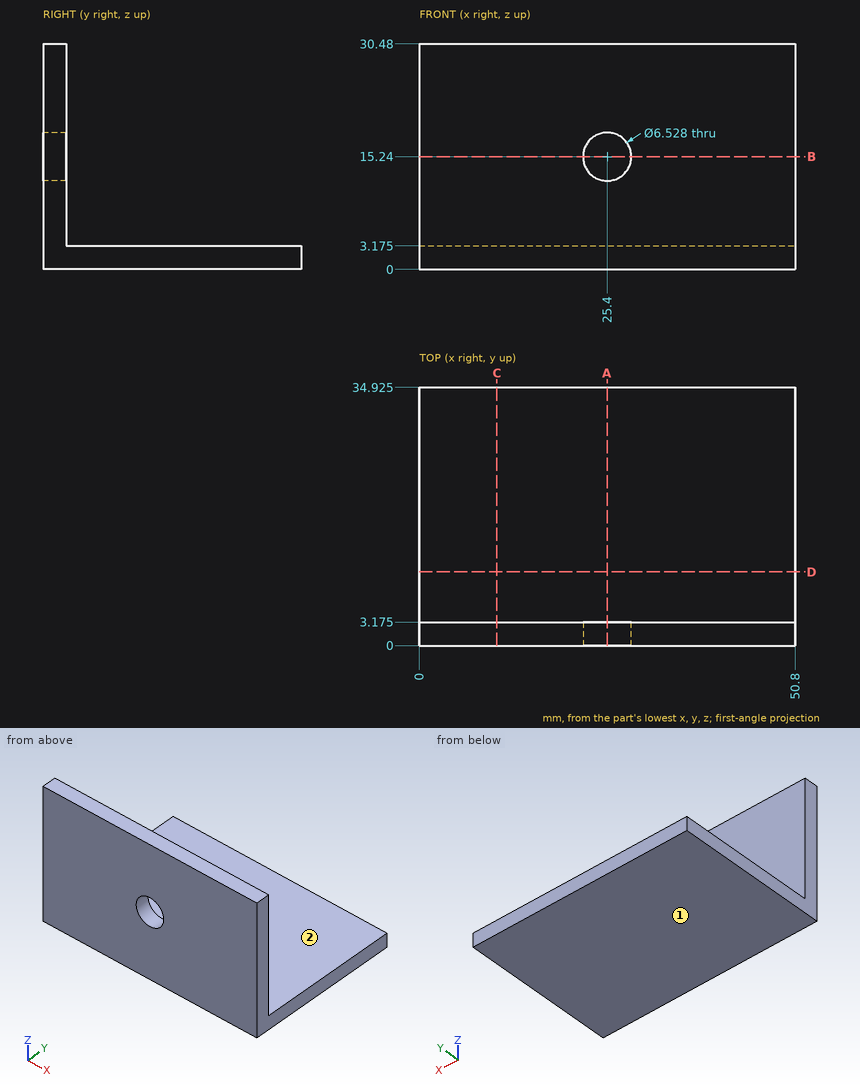
Answer from the drawing. Dimensions are ordinates in mm from the lowest x, y and z of the part. A direction names the side the tool comes from. Give positions to 0.01 mm unless a question says otherwise; leave off trailing zeros. Write each loop counter-clockwise with the first axis right and the second up, starting at its lowest first coordinate (ties: lowest second). Pieces come first, ordered by that corner, then holes. Notation, with made-up numbers: (22, -11) - (81, -11) arc R28 ccw to (81, 7) - close; hole circle Ø7 at (67, -14.75). An arc over 180 degrees is marked (long way). One line per item, written item: value. Start each with the question number.
1. Find section B-B (z = 15.24). Write down the section's boundary in (x, y) (1 decimal).
2. Given pin 1 (4 mm diameter, centred on x = 25.4, z = 15.24, fed in from -Y); pin 2 (2 mm diameter, centred on x = 37, z = 14.5, fed in from +Y) (3 decimals); pin 3 (1.5 mm diameter, centred on x = 19.5, y = 26.5, fed in from +Z) (3 decimals), each flat-ended and moving along its own axis, determine where each tip first touches the part or whether it passes through.
3. Find section C-C (x = 10.5). Write down the section's boundary in (y, z) (3 decimals).
4. Find section D-D (y = 10). Write down the section's boundary in (x, z) (3 decimals), then the cut area to 3 significant figures.
5. For the marked faces 1 and 2, determine the directions among +Z, -Z, +X, -X, +Y, -Y from which every point of the face is accessible in a straight line to the end or side of a thin tool.
6. Find section A-A (x = 25.4). Write down the section's boundary in (y, z) (1 decimal), then the cut area to 3 significant figures.
7. Consider probe 1 along Z at (x, y) = (25.4, 2.15); probe 2 along X at (y, z) = (2, 15) (1 decimal); probe 3 along Y at (x, z) = (37, 7.5) (3 decimals). Determine where each line is inside the solid, lowest interval first.
Geometry results:
1. outline: (0, 0) - (22.1, 0) - (22.1, 3.2) - (0, 3.2) - close; (28.7, 0) - (50.8, 0) - (50.8, 3.2) - (28.7, 3.2) - close
2. pin 1: through
2. pin 2: y = 3.175
2. pin 3: z = 3.175
3. outline: (0, 0) - (34.925, 0) - (34.925, 3.175) - (3.175, 3.175) - (3.175, 30.48) - (0, 30.48) - close
4. outline: (0, 0) - (50.8, 0) - (50.8, 3.175) - (0, 3.175) - close
4. area: 161 mm2
5. face 1: -Z, +X, -X, +Y, -Y
5. face 2: +Z, +X, -X, +Y
6. outline: (0, 0) - (34.9, 0) - (34.9, 3.2) - (3.2, 3.2) - (3.2, 12) - (0, 12) - close; (0, 18.5) - (3.2, 18.5) - (3.2, 30.5) - (0, 30.5) - close
6. area: 177 mm2
7. probe 1: 0 to 11.98, 18.5 to 30.48
7. probe 2: 0 to 22.1, 28.7 to 50.8
7. probe 3: 0 to 3.175
